Could you check a few things on this model? Use its own coordinates, in mm. A direction names the side the tool comes from. Round coordinates to 2 decimals unless told otherwise and drop trailing zeros. Loops run counter-clockwise (first coordinate to the right, second up) from the corner with the lowest first, then second, coordinate; pieces in that order, holes last. Notation, with made-up numbers: (-34, 58.5) - (-14, 58.5) arc R31 ccw to (-14, 87.5) - close; hole circle Ø1 at (11, -9.5). An arc over 180 degrees is marked (long way). Use one line per item in the form item = value.
```python
from build123d import *
from build123d.topology import SkipClean

# Parameters (mm, degrees)
BOSS_EXTRUDE1_DEPTH = 44.5
SKETCH2_W           = 6
SKETCH2_H           = 12
CUT_EXTRUDE1_DEPTH  = 10
BOSS_EXTRUDE2_DEPTH = 13
CUT_EXTRUDE2_DEPTH  = 13
SKETCH4_W           = 7
SKETCH4_H           = 13
BOSS_EXTRUDE3_DEPTH = 5
SKETCH5_R           = 1.25
CUT_EXTRUDE3_DEPTH  = 81.78056697
SKETCH7_R           = 1.25
CUT_EXTRUDE4_DEPTH  = 10
CUT_EXTRUDE6_DEPTH  = 8
BOSS_EXTRUDE4_DEPTH = 7.5


with BuildPart() as part:
    # Sketch1 → Boss-Extrude1 (new body)
    with BuildSketch(Plane(origin=(0, 0, 0), x_dir=(1, 0, 0), z_dir=(0, 1, 0))):
        Polygon((0, 0), (2.5, 0), (2.5, 11), (56.5, 11), (56.5, 0), (59, 0), (59, 13), (0, 13), align=None)
    extrude(amount=BOSS_EXTRUDE1_DEPTH)

    # Sketch2 → Cut-Extrude1 (cut)
    with BuildSketch(Plane(origin=(59, 0, 0), x_dir=(0, 0, -1), z_dir=(1, 0, 0))):
        with Locations((3, 29)):
            Rectangle(SKETCH2_W, SKETCH2_H)
    extrude(amount=-CUT_EXTRUDE1_DEPTH, mode=Mode.SUBTRACT)

    # Sketch3 → Boss-Extrude2 (add)
    with BuildSketch(Plane(origin=(0, 0, -13), x_dir=(-1, 0, 0), z_dir=(0, 0, -1))):
        with BuildLine():
            Line((-59, 6.145643924), (-59, 8))
            Line((-59, 8), (-59.5, 8))
            ThreePointArc((-59.5, 8), (-62.5, 5), (-59.5, 2))
            Line((-59.5, 2), (-59, 2))
            Line((-59, 2), (-59, 3.854356076))
            ThreePointArc((-59, 3.854356076), (-60.75, 5), (-59, 6.145643924))
        make_face()
        with BuildLine():
            Line((0.5, 8), (0, 8))
            Line((0, 8), (0, 6.145643924))
            ThreePointArc((0, 6.145643924), (1.184653197, 6.045825033), (1.75, 5))
            ThreePointArc((1.75, 5), (1.184653197, 3.954174967), (0, 3.854356076))
            Line((0, 3.854356076), (0, 2))
            Line((0, 2), (0.5, 2))
            ThreePointArc((0.5, 2), (3.5, 5), (0.5, 8))
        make_face()
    extrude(amount=-BOSS_EXTRUDE2_DEPTH)

    # Sketch3_3 → Cut-Extrude2 (cut)
    with SkipClean():  # the faces are left unmerged after this step: merging them gives an invalid solid
        with BuildSketch(Plane(origin=(0, 0, -13), x_dir=(-1, 0, 0), z_dir=(0, 0, -1))):
            with BuildLine():
                ThreePointArc((-58.25, 5), (-58.454174967, 5.684653197), (-59, 6.145643924))
                Line((-59, 6.145643924), (-59, 3.854356076))
                ThreePointArc((-59, 3.854356076), (-58.454174967, 4.315346803), (-58.25, 5))
            make_face()
            with BuildLine():
                Line((-59, 3.854356076), (-59, 6.145643924))
                ThreePointArc((-59, 6.145643924), (-60.75, 5), (-59, 3.854356076))
            make_face()
            with BuildLine():
                ThreePointArc((1.75, 5), (1.184653197, 6.045825033), (0, 6.145643924))
                Line((0, 6.145643924), (0, 3.854356076))
                ThreePointArc((0, 3.854356076), (1.184653197, 3.954174967), (1.75, 5))
            make_face()
            with BuildLine():
                Line((0, 3.854356076), (0, 6.145643924))
                ThreePointArc((0, 6.145643924), (-0.75, 5), (0, 3.854356076))
            make_face()
        extrude(amount=-CUT_EXTRUDE2_DEPTH, mode=Mode.SUBTRACT)

    # Sketch4 → Boss-Extrude3 (add)
    with SkipClean():  # the faces are left unmerged after this step: merging them gives an invalid solid
        with BuildSketch(Plane(origin=(0, 44.5, 0), x_dir=(1, 0, 0), z_dir=(0, 1, 0))):
            with Locations((3.5, 6.5)):
                Rectangle(SKETCH4_W, SKETCH4_H)
            with Locations((55.5, 6.5)):
                Rectangle(SKETCH4_W, SKETCH4_H)
        extrude(amount=BOSS_EXTRUDE3_DEPTH)

    # Sketch5 → Cut-Extrude3 (cut, through all)
    with SkipClean():  # the faces are left unmerged after this step: merging them gives an invalid solid
        with BuildSketch(Plane(origin=(0, 0, -13), x_dir=(-1, 0, 0), z_dir=(0, 0, -1))):
            with Locations((-55.5, 47)):
                Circle(SKETCH5_R)
            with Locations((-3.5, 47)):
                Circle(SKETCH5_R)
            with Locations((-6, 73.35)):
                Circle(SKETCH5_R)
            with Locations((-53, 73.35)):
                Circle(SKETCH5_R)
        extrude(amount=-CUT_EXTRUDE3_DEPTH, mode=Mode.SUBTRACT)

    # Sketch7 → Cut-Extrude4 (cut)
    with SkipClean():  # the faces are left unmerged after this step: merging them gives an invalid solid
        with BuildSketch(Plane(origin=(0, 0, -13), x_dir=(-1, 0, 0), z_dir=(0, 0, -1))):
            with Locations((-53.1, 2.9)):
                Circle(SKETCH7_R)
            with Locations((-5.9, 2.9)):
                Circle(SKETCH7_R)
            with Locations((-53.1, 40.95)):
                Circle(SKETCH7_R)
            with Locations((-5.9, 40.95)):
                Circle(SKETCH7_R)
        extrude(amount=-CUT_EXTRUDE4_DEPTH, mode=Mode.SUBTRACT)

    # Sketch3_4 → Cut-Extrude6 (cut)
    with SkipClean():  # the faces are left unmerged after this step: merging them gives an invalid solid
        with BuildSketch(Plane(origin=(0, 0, -13), x_dir=(-1, 0, 0), z_dir=(0, 0, -1))):
            with BuildLine():
                Line((-59, 6.145643924), (-59, 8))
                Line((-59, 8), (-59.5, 8))
                ThreePointArc((-59.5, 8), (-62.5, 5), (-59.5, 2))
                Line((-59.5, 2), (-59, 2))
                Line((-59, 2), (-59, 3.854356076))
                ThreePointArc((-59, 3.854356076), (-60.75, 5), (-59, 6.145643924))
            make_face()
            with BuildLine():
                Line((0.5, 8), (0, 8))
                Line((0, 8), (0, 6.145643924))
                ThreePointArc((0, 6.145643924), (1.184653197, 6.045825033), (1.75, 5))
                ThreePointArc((1.75, 5), (1.184653197, 3.954174967), (0, 3.854356076))
                Line((0, 3.854356076), (0, 2))
                Line((0, 2), (0.5, 2))
                ThreePointArc((0.5, 2), (3.5, 5), (0.5, 8))
            make_face()
        extrude(amount=-CUT_EXTRUDE6_DEPTH, mode=Mode.SUBTRACT)

    # Sketch3_5 → Boss-Extrude4 (add)
    with SkipClean():  # the faces are left unmerged after this step: merging them gives an invalid solid
        with BuildSketch(Plane(origin=(0, 0, -13), x_dir=(-1, 0, 0), z_dir=(0, 0, -1))):
            with BuildLine():
                Line((0, 3.854356076), (0, 6.145643924))
                ThreePointArc((0, 6.145643924), (-0.75, 5), (0, 3.854356076))
            make_face()
            with BuildLine():
                ThreePointArc((-58.25, 5), (-58.454174967, 5.684653197), (-59, 6.145643924))
                Line((-59, 6.145643924), (-59, 3.854356076))
                ThreePointArc((-59, 3.854356076), (-58.454174967, 4.315346803), (-58.25, 5))
            make_face()
        extrude(amount=-BOSS_EXTRUDE4_DEPTH)


solid = part.part
```
1. If we section it at B-B, the plane x = 55.5: Write out the boundary of the cut face in (y, z).
Solution:
outline = (0, -13) - (45.75, -13) - (45.75, 0) - (44.5, 0) - (44.5, -11) - (0, -11) - close; (48.25, -13) - (49.5, -13) - (49.5, 0) - (48.25, 0) - close
2. If we section it at A-A, the plane y = 40.95: Write out the boundary of the cut face in (x, z), plus the area to 3 significant figures.
Solution:
outline = (0, -13) - (4.65, -13) - (4.65, -11) - (2.5, -11) - (2.5, 0) - (0, 0) - close; (7.15, -13) - (51.85, -13) - (51.85, -11) - (7.15, -11) - close; (54.35, -13) - (59, -13) - (59, 0) - (56.5, 0) - (56.5, -11) - (54.35, -11) - close
area = 163 mm^2
3. We'd pull the mould along Y, two halves only. Please class faces 4 (the face through (52, 47, -6)), 5 (the face through (3, 49.5, -7)), 6 (the face through (58, 35, -3)): +Y half, -Y half, draft (parallel to the pull), parting line (faces both ways), or undercut.
Solution:
face_4 = draft
face_5 = +Y half
face_6 = undercut
4. If we section it at C-C, the plane x = 5.9: Write out the boundary of the cut face in (y, z).
Solution:
outline = (0, -13) - (1.65, -13) - (1.65, -11) - (0, -11) - close; (4.15, -13) - (39.7, -13) - (39.7, -11) - (4.15, -11) - close; (42.2, -13) - (49.5, -13) - (49.5, 0) - (44.5, 0) - (44.5, -11) - (42.2, -11) - close
5. For P1, Ø5.5, axis at y = 47, z = -8, coming from the +X side; P2, Ø1.2, axis at x = 58.5, y = 26, coming from the +Z side; P3, Ø1.5, axis at y = 5.5, z = -6, coming from the -X side; P4, Ø2, axis at x = 3.5, y = 47, coming from the +Z side, each with a flat end and sliding along its axis, tell me the tip position at first contact or that it passes through.
Solution:
P1 = 59
P2 = -6
P3 = 0
P4 = through
6. If we section it at D-D, the plane y = 47: Write out the boundary of the cut face in (x, z).
Solution:
outline = (0, -13) - (2.25, -13) - (2.25, 0) - (0, 0) - close; (4.75, -13) - (7, -13) - (7, 0) - (4.75, 0) - close; (52, -13) - (54.25, -13) - (54.25, 0) - (52, 0) - close; (56.75, -13) - (59, -13) - (59, 0) - (56.75, 0) - close
7. On a 3-axis mill with a long thin cutter (end or side, diameter ignored), from which of +Z, -Z, +X, -X, +Y, -Y can I reach the whole of each face in a straight line? I mean faces 1 (the face through (-2, 5, -5)), 2 (the face through (61, 5, -5)), 3 (the face through (2.5, 22, -5)). Say none if no direction works.
Solution:
face_1 = -Z, -X, +Y, -Y
face_2 = -Z, +X, +Y, -Y
face_3 = +Z, -Y
8. Please list where these lines run through material, in increasing order: line 1 along Y through (x, z) = (5.9, -12.3); line 2 along X through (y, z) = (31.5, -7.25); line 3 along Y through (x, z) = (3.5, -2.5).
Solution:
line_1 = 0 to 1.65, 4.15 to 39.7, 42.2 to 49.5
line_2 = 0 to 2.5, 56.5 to 59
line_3 = 44.5 to 45.75, 48.25 to 49.5
